Verification items for the finished model (mm, model axes). Give positions to 0.01 mm unless a question says otherwise; leave off trailing zeros. Order: outer loops, then holes, each group sorted by start corner. A loop starts at its lowest first (then second) coordinate and runs counter-clockwise, first axis right, second up.
(1) Mould release check, pull along Z, two halves, no side actions. Record for faces 1 (the face through (5.35, 1.48, -46.77)), 2 (the face through (0.6, 1.48, -0.57)), 3 (the face through (0.57, 1.48, -49.4)): pulls with the +Z half, pulls with the -Z half, needs draft (parallel to the pull), parting line crosses it, or undercut.
(2) Sectioned sample at A-A on z = -45. Record the cut outline in (x, y), plus the area to 3 significant figures.
(3) Sectioned sample at B-B on x = 45.5. Record the cut outline in (y, z), plus the area to 3 significant figures.
(4) Scan lines: L1, parallel to Z at x = 4.5, y = 2.35; L2, parallel to X at y = 0.8, z = -46. Record each from-to range of solid material in increasing order.
(5) Gauge pin test, flat end, axial feed: pin 1 (2.5 mm diameter, centred on x = 45.76, z = -45.76, fed in from -Y) (3 decimals). Record the tip position at first contact, or that the pin passes through.
Autodesk Inventor part; units mm, degrees
ref_plane "YZ Plane" through (0, 0, 0) normal (1, 0, 0) x (0, 1, 0)
ref_plane "XZ Plane" through (0, 0, 0) normal (0, 1, 0) x (-1, 0, 0)
ref_plane "XY Plane" through (0, 0, 0) normal (0, 0, 1) x (1, 0, 0)
sketch "Sketch3" plane through (0, 0, 0) normal (0, 1, 0) x (-1, 0, 0)
  line L0 (-15, 0) -> (-2, 0)
  line L1 (0, -2) -> (0, -48)
  line L2 (-2, -50) -> (-48, -50)
  line L3 (-50, -48) -> (-50, -2)
  circle A0 centre (-4.2426, -4.2426) radius 1.5
  circle A1 centre (-4.2426, -45.7574) radius 1.5
  circle A2 centre (-45.7574, -45.7574) radius 1.5
  circle A3 centre (-45.7574, -4.2426) radius 1.5
  line L4 (-35, 0) -> (-48, 0)
  arc A4 (0, -2) -> (-2, 0) centre (-2, -2) ccw
  arc A5 (-48, 0) -> (-50, -2) centre (-48, -2) ccw
  arc A6 (-50, -48) -> (-48, -50) centre (-48, -48) ccw
  arc A7 (-2, -50) -> (0, -48) centre (-2, -48) ccw
  line L5 (-48, 0) -> (-2, 0)
  point P0 (0, 0)
  point P1 (0, 0)
  point P2 (-50, 0)
  point P3 (0, 0)
  point P4 (0, -50)
  dimension "d19" = 50
  dimension "d20" = 50
  dimension "d21" = 3
  dimension "d22" = 3
  dimension "d23" = 3
  dimension "d24" = 3
  dimension "d32" = 2
extrude "Extrusion2" add sketch "Sketch3" along normal blind 3
properties part number "Batt_Plate_FPV"
Ans:
1. face 1: undercut
1. face 2: pulls with the +Z half
1. face 3: pulls with the -Z half
2. outline: (0, 0) - (2.95, 0) - (2.95, 3) - (0, 3) - close; (5.54, 0) - (44.46, 0) - (44.46, 3) - (5.54, 3) - close; (47.05, 0) - (50, 0) - (50, 3) - (47.05, 3) - close
2. area: 134 mm2
3. outline: (0, -50) - (3, -50) - (3, -47.24) - (0, -47.24) - close; (0, -44.28) - (3, -44.28) - (3, -5.72) - (0, -5.72) - close; (0, -2.76) - (3, -2.76) - (3, 0) - (0, 0) - close
3. area: 132 mm2
4. L1: z = -50 to -47.24, -44.28 to -5.72, -2.76 to 0
4. L2: x = 0 to 2.76, 5.72 to 44.28, 47.24 to 50
5. pin 1: passes through
